Verification items for the finished model (mm, model axes). Coordinates: 2 decimals unless noted, no trailing zeros. Write each loop counter-clockwise with the first axis right and the second up, starting at its lowest first coordinate (ties: lowest second). Pieces come first, ordered by that corner, then holes. Notation, with made-up numbers: (60.25, 87) -> (91.25, 87) arc R10 cw to (91.25, 101) -> close; hole circle Ø9 at (37, 32.5). An arc over 180 degrees is marked (long way). Answer in a Markdown table with one row per item.
```python
from build123d import *

# Parameters (mm, degrees)
F0_W         = 16
F0_H         = 16
F1_DEPTH     = 16
F2_R         = 2
F3_T1_DEPTH  = 12
F3_S5_W      = 2
F3_S5_H      = 2
F3_T6_DEPTH  = 2
F3_S11_W     = 2
F3_S11_H     = 2
F3_T12_DEPTH = 2


# Not quite as in the source:
# - a fillet or chamfer that OpenCascade refuses, or shapes differently, is made with other operations: its cross-section is extruded or revolved along the edge and cut away or added


with BuildPart() as f1:
    # F0 (on Front) → F1 (new body)
    with BuildSketch(Plane.XZ):
        Rectangle(F0_W, F0_H)
    extrude(amount=F1_DEPTH)

    # F2
    f2_edges = [f1.edges().sort_by_distance(p)[0] for p in [
        (0, -16, 8),
        (8, -8, 8),
        (8, -8, -8),
        (-8, -16, 0),
        (8, 0, 0),
        (8, -16, 0),
        (-8, -8, -8),
        (-8, -8, 8),
        (-8, 0, 0),
        (0, 0, 8),
        (0, 0, -8),
    ]]
    fillet(f2_edges, radius=F2_R)

    # F3: fillet of radius 2 on 1 edges, made by hand

    # F3_s2 → F3_t1 (cut)
    with BuildSketch(Plane.YZ.offset(-6)):
        with BuildLine():
            ThreePointArc((-16, -6), (-15.4142135624, -7.4142135624), (-14, -8))
            Line((-14, -8), (-16, -8))
            Line((-16, -8), (-16, -6))
        make_face()
    extrude(amount=F3_T1_DEPTH, mode=Mode.SUBTRACT)


with BuildPart() as f3_tool4:
    # F3_s5 → F3_t6 (new body)
    with BuildSketch(Plane.XZ.offset(14)):
        with Locations((-7, -7)):
            Rectangle(F3_S5_W, F3_S5_H)
    extrude(amount=F3_T6_DEPTH)

    # F3_s7 → F3_t8 (revolve, cut)
    with BuildSketch(Plane(origin=(-6, -14, -6), x_dir=(0.7071067812, 0, 0.7071067812), z_dir=(0.7071067812, 0, -0.7071067812))):
        with BuildLine():
            ThreePointArc((0, -2), (2, 0), (0, 2))
            Line((0, 2), (0, -2))
        make_face()
    revolve(axis=Axis((-6, -14, -6), (0, -1, 0)), mode=Mode.SUBTRACT)


with BuildPart() as f1_1:
    add(f1.part)

    # F3_t3: cut F3_tool4
    add(f3_tool4.part, mode=Mode.SUBTRACT)


with BuildPart() as f3_tool10:
    # F3_s11 → F3_t12 (new body)
    with BuildSketch(Plane.XZ.offset(14)):
        with Locations((7, -7)):
            Rectangle(F3_S11_W, F3_S11_H)
    extrude(amount=F3_T12_DEPTH)

    # F3_s13 → F3_t14 (revolve, cut)
    with BuildSketch(Plane(origin=(6, -14, -6), x_dir=(-0.7071067812, 0, 0.7071067812), z_dir=(0.7071067812, 0, 0.7071067812))):
        with BuildLine():
            ThreePointArc((0, -2), (2, 0), (0, 2))
            Line((0, 2), (0, -2))
        make_face()
    revolve(axis=Axis((6, -14, -6), (0, -1, 0)), mode=Mode.SUBTRACT)


with BuildPart() as f1_2:
    add(f1_1.part)

    # F3_t9: cut F3_tool10
    add(f3_tool10.part, mode=Mode.SUBTRACT)


solid = f1_2.part
```
1. Section check A-A, the plane z = 6.75. Record the boundary of the cut face in (x, y).
Geometry says:
| item | result |
|---|---|
| outline | (-7.85, -14) arc R1.85 ccw to (-6, -15.85) -> (6, -15.85) arc R1.85 ccw to (7.85, -14) -> (7.85, -2) arc R1.85 ccw to (6, -0.15) -> (-6, -0.15) arc R1.85 ccw to (-7.85, -2) -> close |
2. Section check B-B, the plane y = -1.5. Record the boundary of the cut face in (x, z).
Geometry says:
| item | result |
|---|---|
| outline | (-7.94, -6) arc R1.94 ccw to (-6, -7.94) -> (6, -7.94) arc R1.94 ccw to (7.94, -6) -> (7.94, 6) arc R1.94 ccw to (6, 7.94) -> (-6, 7.94) arc R1.94 ccw to (-7.94, 6) -> close |
3. Thickness scan on line 1 (Y direction, x = 6.5, z = 6); line 2 (Y direction, x = 5.25, z = -7.5); line 3 (X direction, y = -10.25, z = -7.5). Record the ranges inside material, lowest first. Write a range as from..to.
Geometry says:
| item | result |
|---|---|
| line 1 | -15.94..-0.06 |
| line 2 | -15.32..-0.68 |
| line 3 | -7.32..7.32 |
4. Depth check by flat-ended pin: P1, Ø1, axis at x = 0, z = 3, coming from the +Y side. Enter the tip coordinate at first touch or a pass-through.
Geometry says:
| item | result |
|---|---|
| P1 | y = 0 |
